For this review, take the finished solid that the model builds, in its own axes (mm). Face numbers are marked on the shaded views. Round coordinates to 2 decimals unless told otherwise and drop trailing zeros. Write each loop counter-clockwise with the first axis right and the second up, starting at its lowest first coordinate (ties: lowest second). Pieces come first, ordered by that corner, then holes. Notation, with made-up numbers: (-12, -38.75) - (38, -38.75) arc R23 ccw to (38, -27.75) - close; hole circle Ø7 at (3.25, 78). An arc over 180 degrees is marked (long way). One line per item, written item: value. Start each with the question number.
Q1. For probe 1 along X at (y, z) = (34, 2.8); probe 2 along Y at (x, z) = (21, 2.3); probe 3 along Z at (x, y) = (-18, 47), list the stretches that pass through material, from the lowest coordinate up.
Q2. Clearance check with a flat-ended pin moving along its axis: pin 1 Ø12 at (x, y) = (-1.5, 4) entering from +Z. State where the tip first meets the part, or that it passes through.
Q3. Add section A-A on z = 0.8. Write out the cut boundary in (x, y), and give its area (3 significant figures).
Q4. Add section C-C on x = -52. Write out the cut boundary in (y, z).
Q5. Mouldability with a two-part tool opening along Y and no side actions: class the marked faces 1 and 2 as +Y half, -Y half, draft (parallel to the pull), parting line (faces both ways), or undercut.
Q6. Add section B-B on y = 33.5. Write out the cut boundary in (x, z).
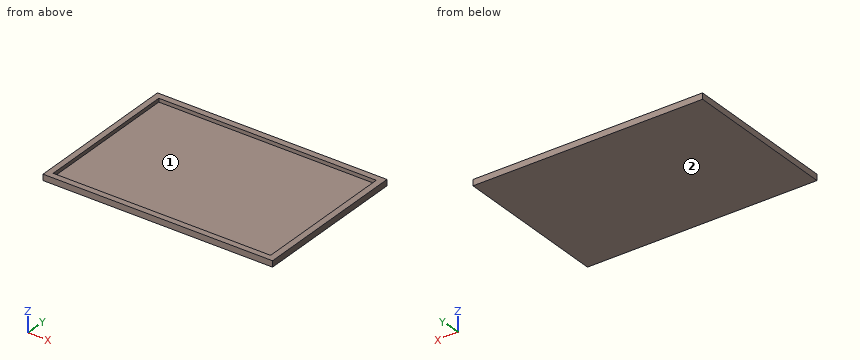
```python
from build123d import *

# Parameters (mm, degrees)
SKETCH_W     = 160
SKETCH_H     = 100
PAD_DEPTH    = 2
SKETCH001_W  = 180
SKETCH001_H  = 120
PAD001_DEPTH = 5
SKETCH006_W  = 190
SKETCH006_H  = 130
PAD006_DEPTH = 5


with BuildPart() as pcb:
    # Sketch → Pad (new body)
    with BuildSketch(Plane(origin=(-1, 1, 3), x_dir=(1, 0, 0), z_dir=(0, 0, 1))):
        with Locations((11.269221, -1.548084)):
            Rectangle(SKETCH_W, SKETCH_H)
    extrude(amount=PAD_DEPTH)


with BuildPart() as portapcb001:
    # Sketch001 → Pad001 (new body)
    with BuildSketch(Plane.XY):
        with Locations((9.825213, -0.104076)):
            Rectangle(SKETCH001_W, SKETCH001_H)
    extrude(amount=PAD001_DEPTH)

    # Cut001: cut PCB
    add(pcb.part, mode=Mode.SUBTRACT)


with BuildPart() as base:
    # Sketch006 → Pad006 (new body)
    with BuildSketch(Plane.XY.offset(-2)):
        with Locations((10, 0)):
            Rectangle(SKETCH006_W, SKETCH006_H)
    extrude(amount=PAD006_DEPTH)

    # Cut002: cut PortaPCB001
    add(portapcb001.part, mode=Mode.SUBTRACT)


solid = base.part
```
Result set:
1. probe 1: x = -85 to -80.17, 99.83 to 105
1. probe 2: y = -65 to -60.1, 59.9 to 65
1. probe 3: z = -2 to 0
2. pin 1: stops at z = 0
3. outline: (-85, -65) - (105, -65) - (105, 65) - (-85, 65) - close; hole (-80.17, -60.1) - (99.83, -60.1) - (99.83, 59.9) - (-80.17, 59.9) - close
3. area: 3,100 mm^2
4. outline: (-65, -2) - (65, -2) - (65, 3) - (59.9, 3) - (59.9, 0) - (-60.1, 0) - (-60.1, 3) - (-65, 3) - close
5. face 1: undercut
5. face 2: draft
6. outline: (-85, -2) - (105, -2) - (105, 3) - (99.83, 3) - (99.83, 0) - (-80.17, 0) - (-80.17, 3) - (-85, 3) - close
